For this review, use the dimensioned drawing (mm, ordinates from the lowest corner) and the shaded views. A direction names the side the tool comes from. Round coordinates to 2 decimals unless told otherwise and drop trailing zeros. Order: outer loops, then holes, each group sorted by start corner. A loop starts at its lowest first (then second) coordinate and runs counter-clockwise, first axis right, second up. Notation, with made-up numbers: M 41,89 L 87,89 A21 cw 87,100 Z; hole C 15,21 d7. An arc over 180 degrees is marked long. One line per item, written item: value. Start each with the question number.
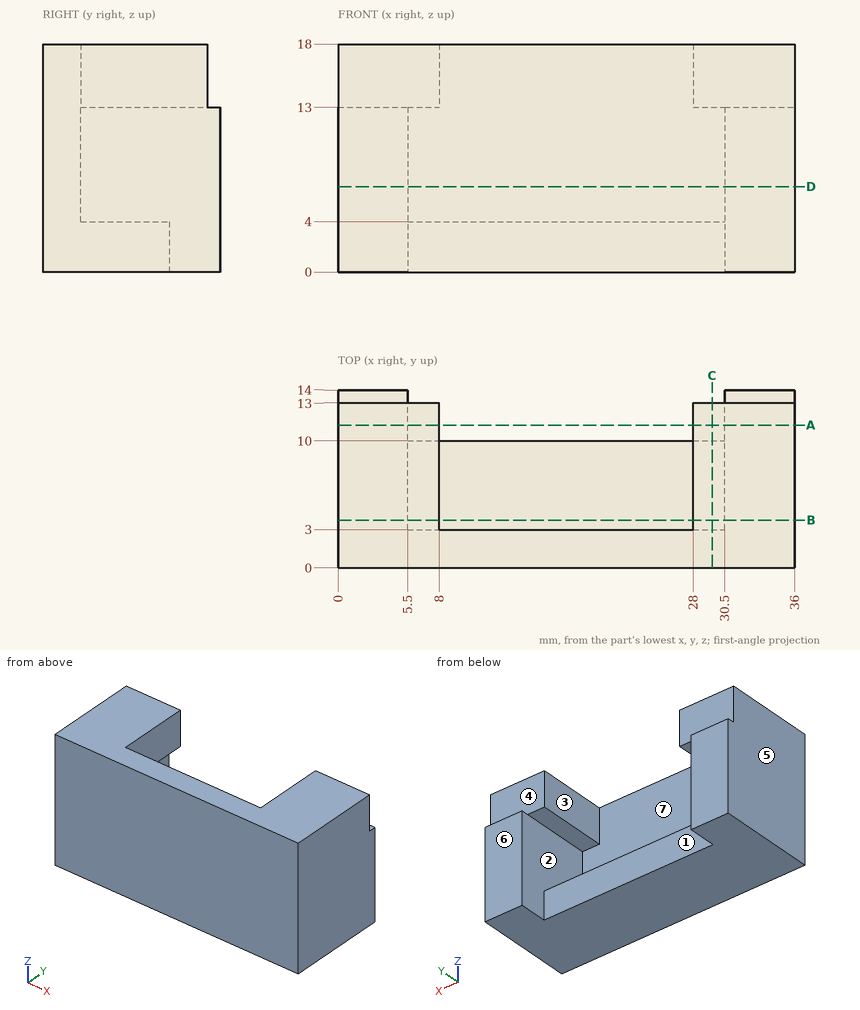
Item 1: Consider section A-A, the plane y = 11.25. Give the boundary of the cut face in (x, z).
Item 2: Wall thickness on L1, parallel to X at y = 7.25, z = 7.25; L2, parallel to Z at x = 29.5, y = 5; L3, parallel to Z at x = 26, y = 8.5: over which ranges is each line inside the solid? List them lowest first.
Item 3: Clearance check with flat-ended pins moving along their axes: P1, Ø4, axis at y = 12.5, z = 4, coming from the -X side; P2, Ø1.5, axis at x = 23, z = 5, coming from the +Y side; P3, Ø8, axis at x = 15.5, z = 4, coming from the +Y side; P4, Ø5.5, axis at x = 31.5, z = 16.5, coming from the +Y side. State where each tip first meets the part, or that it passes through.
Item 4: Machinability: for the marked faces 1, 2, 3 and 4, which of the approach directions +Z, -Z, +X, -X, +Y, -Y give a long, thin tool a straight path to every point of the face, cutting with its end or side? Answer none if there is none.
Item 5: The part is to be moulded in two halves that separate along X. For the marked faces 5, 6 and 7, say which applies: pulls with the +X half, pulls with the -X half, needs draft (parallel to the pull), parting line crosses it, or undercut.
Item 6: Consider section D-D, the plane z = 6.75. Give the boundary of the cut face in (x, y), then the cut area to 3 significant figures.
Item 7: Consider section C-C, the plane x = 29.5. Give the boundary of the cut face in (y, z), then the cut area to 3 significant figures.
Item 8: Consider section B-B, the plane y = 3.75. Give the boundary of the cut face in (x, z).
Computed:
1. outline: M 0,0 L 5.5,0 L 5.5,13 L 8,13 L 8,18 L 0,18 Z; M 28,13 L 30.5,13 L 30.5,0 L 36,0 L 36,18 L 28,18 Z
2. L1: x = 0 to 5.5, 30.5 to 36
2. L2: z = 0 to 4, 13 to 18
2. L3: z = 0 to 4
3. P1: stops at x = 0
3. P2: stops at y = 3
3. P3: stops at y = 10
3. P4: stops at y = 13
4. face 1: -Z, +Y
4. face 2: +Y
4. face 3: +Z, +Y
4. face 4: +Z, +X, -X, +Y
5. face 5: pulls with the -X half
5. face 6: needs draft
5. face 7: undercut
6. outline: M 0,0 L 36,0 L 36,14 L 30.5,14 L 30.5,3 L 5.5,3 L 5.5,14 L 0,14 Z
6. area: 229 mm^2
7. outline: M 0,0 L 10,0 L 10,4 L 3,4 L 3,13 L 13,13 L 13,18 L 0,18 Z
7. area: 132 mm^2
8. outline: M 0,0 L 36,0 L 36,18 L 28,18 L 28,13 L 30.5,13 L 30.5,4 L 5.5,4 L 5.5,13 L 8,13 L 8,18 L 0,18 Z
